Here's the drawing with two shaded views (mm, measured from the low corner). I have some questions. Round coordinates to 2 decimals unless told otherwise and drop trailing zeros. Order: outer loops, then holes, each group sorted by start corner. A loop starts at its lowest first (then second) coordinate and runs counter-clockwise, first axis right, second up.
Q1. If I drill on line 1 (X direction, y = 43, z = 43); line 2 (Z direction, x = 204.5, y = 21), over which ranges is the centre line in solid material (lowest first)?
Q2. We'd pull the mould along X, two halves only. Please class the marked faces 1, 2, 3 and 4: pulls with the +X half, pulls with the -X half, needs draft (parallel to the pull), parting line crosses it, or undercut.
Q3. If we section it at A-A (y = 40.5): Please give me the cut outline in (x, z), plus the area to 3 significant figures.
Q4. If we section it at C-C (z = 24.5): Please give me the cut outline in (x, y), plus the area to 3 significant figures.
Q5. Will these pins go through, and if not, where does the flat tip stop? P1, Ø2, axis at x = 221, y = 18.5, coming from the -Z side; P2, Ø8, axis at x = 215.5, z = 16.5, coming from the -Y side; P3, Ø11, axis at x = 118, y = 25.5, coming from the -Z side; P4, Ø5, axis at x = 189.5, z = 24, coming from the +Y side.
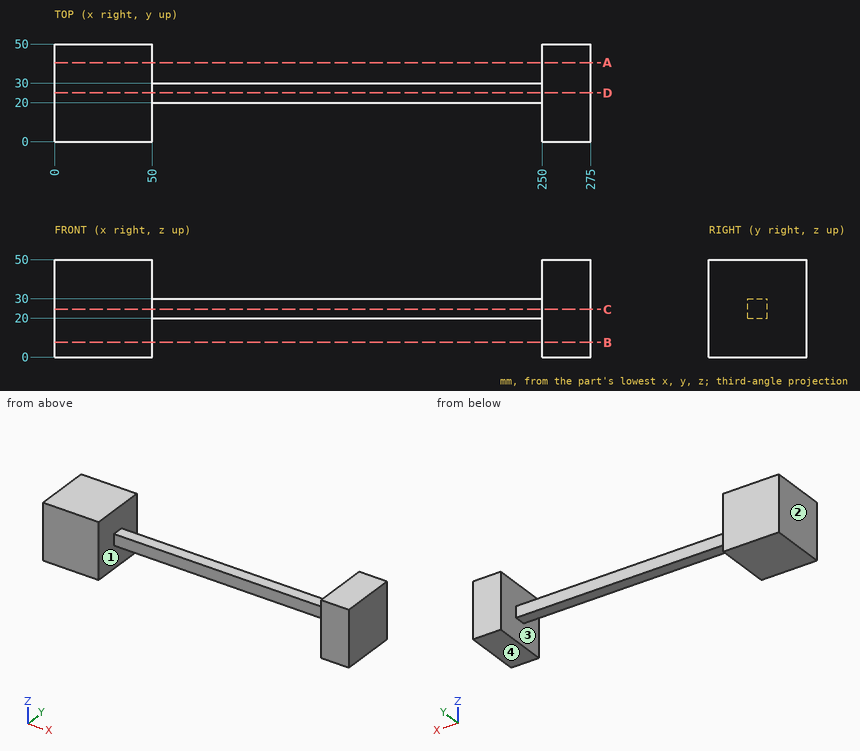
Solution:
1. line 1: x = 0 to 50, 250 to 275
1. line 2: z = 20 to 30
2. face 1: undercut
2. face 2: pulls with the -X half
2. face 3: undercut
2. face 4: needs draft
3. outline: (0, 0) - (50, 0) - (50, 50) - (0, 50) - close; (250, 0) - (275, 0) - (275, 50) - (250, 50) - close
3. area: 3,750 mm2
4. outline: (0, 0) - (50, 0) - (50, 20) - (250, 20) - (250, 0) - (275, 0) - (275, 50) - (250, 50) - (250, 30) - (50, 30) - (50, 50) - (0, 50) - close
4. area: 5,750 mm2
5. P1: passes through
5. P2: stops at y = 20
5. P3: stops at z = 20
5. P4: stops at y = 30
